```python
from build123d import *

# Parameters (mm, degrees)
SKETCH1_W           = 120
SKETCH1_H           = 120
SKETCH1_R           = 57.5
BOSS_EXTRUDE1_DEPTH = 25
FILLET1_R           = 4
SKETCH3_R           = 2
CUT_EXTRUDE1_DEPTH  = 26
BOSS_EXTRUDE2_DEPTH = 3


with BuildPart() as part:
    # Sketch1 → Boss-Extrude1 (new body)
    with BuildSketch(Plane.XY):
        Rectangle(SKETCH1_W, SKETCH1_H)
        Circle(SKETCH1_R, mode=Mode.SUBTRACT)
    extrude(amount=BOSS_EXTRUDE1_DEPTH)

    # Fillet1
    fillet1_edges = [part.edges().sort_by_distance(p)[0] for p in [
        (-60, 60, 12.5),
        (60, 60, 12.5),
        (60, -60, 12.5),
        (-60, -60, 12.5),
    ]]
    fillet(fillet1_edges, radius=FILLET1_R)

    # Sketch2 → Cut-Revolve1 (revolve, cut)
    with BuildSketch(Plane(origin=(0, 0, 0), x_dir=(1, 0, 0), z_dir=(0, 1, 0))):
        Polygon((61, -8.75), (61, -16.25), (65.5, -20.75), (86, -20.75), (86, -4.25), (65.5, -4.25), align=None)
    revolve(axis=Axis((0, 0, 0), (0, 0, 1)), mode=Mode.SUBTRACT)

    # Sketch3 → Cut-Extrude1 (cut, through all)
    with BuildSketch(Plane(origin=(0, 0, 0), x_dir=(-1, 0, 0), z_dir=(0, 0, -1))):
        with Locations((-53.171572875, 53.171572875)):
            Circle(SKETCH3_R)
        with Locations((53.171572875, 53.171572875)):
            Circle(SKETCH3_R)
        with Locations((53.171572875, -53.171572875)):
            Circle(SKETCH3_R)
        with Locations((-53.171572875, -53.171572875)):
            Circle(SKETCH3_R)
    extrude(amount=-CUT_EXTRUDE1_DEPTH, mode=Mode.SUBTRACT)

    # Sketch4 → Boss-Extrude2 (add)
    with BuildSketch(Plane.XY.offset(25)):
        with BuildLine():
            ThreePointArc((0, 21), (-9.310739966, 18.823127298), (-16.691166059, 12.743821075))
            ThreePointArc((-16.691166059, 12.743821075), (-0.598422961, 39.925677295), (29.560959215, 49.319364252))
            ThreePointArc((29.560959215, 49.319364252), (25.795909203, 51.388919704), (21.886841663, 53.171572875))
            ThreePointArc((21.886841663, 53.171572875), (-10.667756929, 35.547780517), (-21, 0))
            ThreePointArc((-21, 0), (-18.823127298, -9.310739966), (-12.743821075, -16.691166059))
            ThreePointArc((-12.743821075, -16.691166059), (-39.925677295, -0.598422961), (-49.319364252, 29.560959215))
            ThreePointArc((-49.319364252, 29.560959215), (-51.388919704, 25.795909203), (-53.171572875, 21.886841663))
            ThreePointArc((-53.171572875, 21.886841663), (-35.547780517, -10.667756929), (0, -21))
            ThreePointArc((0, -21), (9.310739966, -18.823127298), (16.691166059, -12.743821075))
            ThreePointArc((16.691166059, -12.743821075), (0.598422961, -39.925677295), (-29.560959215, -49.319364252))
            ThreePointArc((-29.560959215, -49.319364252), (-25.795909203, -51.388919704), (-21.886841663, -53.171572875))
            ThreePointArc((-21.886841663, -53.171572875), (10.667756929, -35.547780517), (21, 0))
            ThreePointArc((21, 0), (18.823127298, 9.310739966), (12.743821075, 16.691166059))
            ThreePointArc((12.743821075, 16.691166059), (39.925677295, 0.598422961), (49.319364252, -29.560959215))
            ThreePointArc((49.319364252, -29.560959215), (51.388919704, -25.795909203), (53.171572875, -21.886841663))
            ThreePointArc((53.171572875, -21.886841663), (35.547780517, 10.667756929), (0, 21))
        make_face()
    extrude(amount=-BOSS_EXTRUDE2_DEPTH)


solid = part.part
```
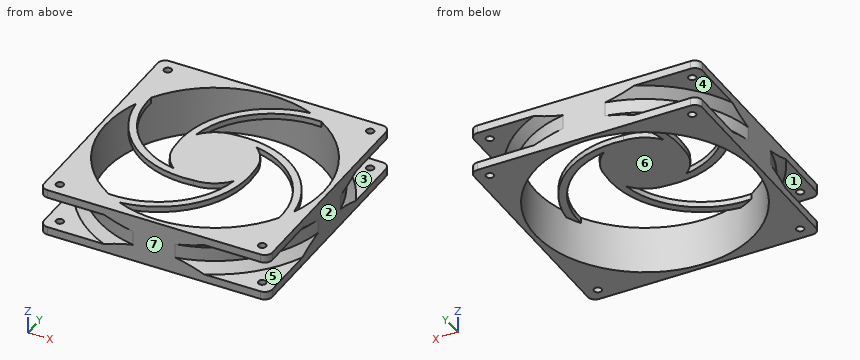
Can you work these out from the model? Positions are in its coordinate system, mm. Face numbers are marked on the shaded views. A direction names the side the tool comes from. Round coordinates to 2 decimals unless told otherwise and drop trailing zeros. Order: outer loops, then holes, each group sorted by start corner. A loop starts at its lowest first (then second) coordinate and runs counter-clockwise, first axis right, second up.
(1) If we section it at C-C (z = 13.75): Please give me the cut outline in (x, y).
Results are:
outline: (-60, -11) arc R61 ccw to (-11, -60) - (11, -60) arc R61 ccw to (60, -11) - (60, 11) arc R61 ccw to (11, 60) - (-11, 60) arc R61 ccw to (-60, 11) - close; hole circle Ø115 at (0, 0)
(2) We'd pull the mould along Y, two halves only. Please class the marked faces 5, 6 and 7: +Y half, -Y half, draft (parallel to the pull), parting line (faces both ways), or undercut.
Results are:
face 5: draft
face 6: undercut
face 7: -Y half
(3) If I drill on L1, parallel to Z at x = 41.5, y = -52; L2, parallel to X at y = 27, z = 23.5; L3, parallel to Z at x = 14, y = 9, over which ranges is the centre line in solid material (lowest first)?
Results are:
L1: z = 0 to 4.25, 20.75 to 25
L2: x = -60 to -49.41, -16.18 to -11.65, 50.77 to 60
L3: z = 22 to 25
(4) On a 3-axis mill with a long thin cutter (end or side, diameter ignored), from which of +Z, -Z, +X, -X, +Y, -Y can I reach the whole of each face in a straight line? I mean the marked faces 1, 2, 3 and 4. Say none if no direction works.
Results are:
face 1: -X, -Y
face 2: +Z, -Z, +X, +Y, -Y
face 3: +X, +Y
face 4: -X, +Y
(5) If we section it at A-A (z = 2): Please give me the cut outline in (x, y), plus the area to 3 significant figures.
Results are:
outline: (-60, -56) arc R4 ccw to (-56, -60) - (56, -60) arc R4 ccw to (60, -56) - (60, 56) arc R4 ccw to (56, 60) - (-56, 60) arc R4 ccw to (-60, 56) - close; hole circle Ø115 at (0, 0); hole circle Ø4 at (-53.17, -53.17); hole circle Ø4 at (-53.17, 53.17); hole circle Ø4 at (53.17, -53.17); hole circle Ø4 at (53.17, 53.17)
area: 3,950 mm2
(6) I'm going to push flat-ended pins straight in: pin 1 (4 mm diameter, centred on x = 17, z = 10, fed in from -Y); pin 2 (6.5 mm diameter, centred on x = 53.17, y = -53.17, fed in from +Z); pin 3 (2 mm diameter, centred on y = 36.5, z = 13, fed in from +X); pin 4 (2 mm diameter, centred on x = -16.5, y = 26, fed in from -Z). Where does each tip first touch, or does it pass through?
Results are:
pin 1: stops at y = -59.44
pin 2: stops at z = 25
pin 3: stops at x = 49.61
pin 4: stops at z = 22
(7) If we section it at B-B (y = 2.5): Please give me the cut outline in (x, z), plus the area to 3 significant figures.
Results are:
outline: (-60, 0) - (-57.45, 0) - (-57.45, 25) - (-60, 25) - close; (-46.87, 22) - (-42.16, 22) - (-42.16, 25) - (-46.87, 25) - close; (-21.22, 22) - (20.85, 22) - (20.85, 25) - (-21.22, 25) - close; (38.33, 22) - (43.51, 22) - (43.51, 25) - (38.33, 25) - close; (57.45, 0) - (60, 0) - (60, 25) - (57.45, 25) - close
area: 284 mm2
